```python
from build123d import *

# Parameters (mm, degrees)
F0_W     = 16.72
F0_H     = 16.25
F0_W_2   = 35.74
F0_H_2   = 18.81
F0_H_3   = 37.3
F0_H_4   = 10.6
F0_W_3   = 16.7007
F1_DEPTH = 4


with BuildPart() as f1:
    # F0 (on Top) → F1 (new body)
    with BuildSketch(Plane.XY):
        Polygon((26.290441, -42.578733), (26.290441, 85.421267), (-128.249559, 85.421267), (-128.249559, 78.421267), (-128.249559, -35.578733), (-128.249559, -42.578733), align=None)
        with Locations((-114.889559, -23.453733)):
            Rectangle(F0_W, F0_H, mode=Mode.SUBTRACT)
        with Locations((-95.869559, -23.453733)):
            Rectangle(F0_W, F0_H, mode=Mode.SUBTRACT)
        with Locations((-76.849559, -23.453733)):
            Rectangle(F0_W, F0_H, mode=Mode.SUBTRACT)
        with Locations((-95.869559, -4.903733)):
            Rectangle(F0_W, F0_H, mode=Mode.SUBTRACT)
        with Locations((-40.619559, -22.083733)):
            Rectangle(F0_W_2, F0_H_2, mode=Mode.SUBTRACT)
        with Locations((-12.089559, -22.083733)):
            Rectangle(F0_W, F0_H_2, mode=Mode.SUBTRACT)
        with Locations((6.930441, -12.778733)):
            Rectangle(F0_W, F0_H_3, mode=Mode.SUBTRACT)
        with Locations((-50.129559, -2.253733)):
            Rectangle(F0_W, F0_H, mode=Mode.SUBTRACT)
        with Locations((-31.109559, -2.253733)):
            Rectangle(F0_W, F0_H, mode=Mode.SUBTRACT)
        with Locations((-50.129559, 16.296267)):
            Rectangle(F0_W, F0_H, mode=Mode.SUBTRACT)
        with Locations((-31.109559, 16.296267)):
            Rectangle(F0_W, F0_H, mode=Mode.SUBTRACT)
        with Locations((-12.089559, -2.253733)):
            Rectangle(F0_W, F0_H, mode=Mode.SUBTRACT)
        with Locations((-12.089559, 16.296267)):
            Rectangle(F0_W, F0_H, mode=Mode.SUBTRACT)
        with Locations((6.930441, 16.296267)):
            Rectangle(F0_W, F0_H, mode=Mode.SUBTRACT)
        with Locations((-114.889559, 34.846267)):
            Rectangle(F0_W, F0_H, mode=Mode.SUBTRACT)
        with Locations((-95.869559, 34.846267)):
            Rectangle(F0_W, F0_H, mode=Mode.SUBTRACT)
        with Locations((-114.889559, 53.396267)):
            Rectangle(F0_W, F0_H, mode=Mode.SUBTRACT)
        with Locations((-95.869559, 53.396267)):
            Rectangle(F0_W, F0_H, mode=Mode.SUBTRACT)
        with Locations((-76.849559, 34.846267)):
            Rectangle(F0_W, F0_H, mode=Mode.SUBTRACT)
        with Locations((-76.849559, 53.396267)):
            Rectangle(F0_W, F0_H, mode=Mode.SUBTRACT)
        with Locations((-114.849559, 69.121267)):
            Rectangle(F0_W, F0_H_4, mode=Mode.SUBTRACT)
        with Locations((-95.849559, 69.121267)):
            Rectangle(F0_W, F0_H_4, mode=Mode.SUBTRACT)
        with Locations((-76.849559, 69.121267)):
            Rectangle(F0_W, F0_H_4, mode=Mode.SUBTRACT)
        with Locations((-50.129559, 34.846267)):
            Rectangle(F0_W, F0_H, mode=Mode.SUBTRACT)
        with Locations((-31.109559, 34.846267)):
            Rectangle(F0_W, F0_H, mode=Mode.SUBTRACT)
        with Locations((-50.129559, 53.396267)):
            Rectangle(F0_W, F0_H, mode=Mode.SUBTRACT)
        with Locations((-31.109559, 53.396267)):
            Rectangle(F0_W, F0_H, mode=Mode.SUBTRACT)
        with Locations((-12.089559, 34.846267)):
            Rectangle(F0_W, F0_H, mode=Mode.SUBTRACT)
        with Locations((6.930441, 34.846267)):
            Rectangle(F0_W, F0_H, mode=Mode.SUBTRACT)
        with Locations((-12.089559, 53.396267)):
            Rectangle(F0_W, F0_H, mode=Mode.SUBTRACT)
        with Locations((6.930441, 53.396267)):
            Rectangle(F0_W, F0_H, mode=Mode.SUBTRACT)
        with Locations((-50.139209, 69.121267)):
            Rectangle(F0_W_3, F0_H_4, mode=Mode.SUBTRACT)
        with Locations((-31.139209, 69.121267)):
            Rectangle(F0_W_3, F0_H_4, mode=Mode.SUBTRACT)
        with Locations((-12.139209, 69.121267)):
            Rectangle(F0_W_3, F0_H_4, mode=Mode.SUBTRACT)
        with Locations((6.860791, 69.121267)):
            Rectangle(F0_W_3, F0_H_4, mode=Mode.SUBTRACT)
    extrude(amount=F1_DEPTH)


solid = f1.part
```
Geometry check sheet. Reference: the model listing, model coordinates, mm. Round coordinates to 2 decimals unless told otherwise and drop trailing zeros. Loops run counter-clockwise (first coordinate to the right, second up) from the corner with the lowest first, then second, coordinate; pieces in that order, holes last. Notation, with made-up numbers: (-34.5, 57.25) - (-21.5, 57.25) arc R31 cw to (-21.5, 84.25) - close; hole circle Ø6 at (-26.5, 60.5). An arc over 180 degrees is marked (long way). Write each question's results on one line, items separated by ' | '. Start each with the question number.
Q1. Cross-section at A-A on y = -17.5. Enter the section's corners in (x, z), and give its area (3 significant figures).
Q2. Cross-section at C-C on x = -93.5. Enter the section's corners in (y, z).
Q3. Cross-section at D-D on y = 16. Enter the section's corners in (x, z).
Q4. Cross-section at B-B on x = -70.5. Enter the section's corners in (y, z).
Q5. Gauge pin test, flat end, axial feed: P1, Ø4, axis at x = -60, y = 47.5, coming from the -Z side. Record the tip position at first contact, or that the pin passes through.
Q6. Thickness scan on line 1 (X direction, y = 23, z = 1.35); line 2 (Y direction, x = -110, z = 0.9); line 3 (Y direction, x = -92, z = 0.4). Record the ranges inside material, lowest first. Write a range as [from, to].
Answers below:
1) outline: (-128.25, 0) - (-123.25, 0) - (-123.25, 4) - (-128.25, 4) - close; (-106.53, 0) - (-104.23, 0) - (-104.23, 4) - (-106.53, 4) - close; (-87.51, 0) - (-85.21, 0) - (-85.21, 4) - (-87.51, 4) - close; (-68.49, 0) - (-58.49, 0) - (-58.49, 4) - (-68.49, 4) - close; (-22.75, 0) - (-20.45, 0) - (-20.45, 4) - (-22.75, 4) - close; (-3.73, 0) - (-1.43, 0) - (-1.43, 4) - (-3.73, 4) - close; (15.29, 0) - (26.29, 0) - (26.29, 4) - (15.29, 4) - close | area: 141 mm²
2) outline: (-42.58, 0) - (-31.58, 0) - (-31.58, 4) - (-42.58, 4) - close; (-15.33, 0) - (-13.03, 0) - (-13.03, 4) - (-15.33, 4) - close; (3.22, 0) - (26.72, 0) - (26.72, 4) - (3.22, 4) - close; (42.97, 0) - (45.27, 0) - (45.27, 4) - (42.97, 4) - close; (61.52, 0) - (63.82, 0) - (63.82, 4) - (61.52, 4) - close; (74.42, 0) - (85.42, 0) - (85.42, 4) - (74.42, 4) - close
3) outline: (-128.25, 0) - (-58.49, 0) - (-58.49, 4) - (-128.25, 4) - close; (-41.77, 0) - (-39.47, 0) - (-39.47, 4) - (-41.77, 4) - close; (-22.75, 0) - (-20.45, 0) - (-20.45, 4) - (-22.75, 4) - close; (-3.73, 0) - (-1.43, 0) - (-1.43, 4) - (-3.73, 4) - close; (15.29, 0) - (26.29, 0) - (26.29, 4) - (15.29, 4) - close
4) outline: (-42.58, 0) - (-31.58, 0) - (-31.58, 4) - (-42.58, 4) - close; (-15.33, 0) - (26.72, 0) - (26.72, 4) - (-15.33, 4) - close; (42.97, 0) - (45.27, 0) - (45.27, 4) - (42.97, 4) - close; (61.52, 0) - (63.82, 0) - (63.82, 4) - (61.52, 4) - close; (74.42, 0) - (85.42, 0) - (85.42, 4) - (74.42, 4) - close
5) P1: stops at z = 0
6) line 1: x = [-128.25, -58.49], [-41.77, -39.47], [-22.75, -20.45], [-3.73, -1.43], [15.29, 26.29] | line 2: y = [-42.58, -31.58], [-15.33, 26.72], [42.97, 45.27], [61.52, 63.82], [74.42, 85.42] | line 3: y = [-42.58, -31.58], [-15.33, -13.03], [3.22, 26.72], [42.97, 45.27], [61.52, 63.82], [74.42, 85.42]
